Source: CAD feature listing. Evaluate the final solid. Frame: model axes, mm. A direction names the side the tool comes from. Give positions to 0.01 mm unless a question says otherwise; leave off trailing zeros. Order: outer loops, then holes, each group sorted by start corner. A loop starts at its lowest first (then second) coordinate and runs counter-clockwise, first axis right, second up. Notation, with made-up numbers: M -14,13.5 L 31,13.5 A21 ccw 31,40.5 Z; hole C -38.75,40.5 d9. An arc over 180 degrees is marked long. Answer in a Markdown table with one row per item. Add a question column.
(1) Set-up query: faces 5 (the face through (6.356, 8.801, 0.279)), 6 (the face through (15.12, 1.25, 11.59)). Return all of +Z, -Z, +X, -X, +Y, -Y with unobstructed straight access to the full face (end or side cutting, diameter ignored); none if empty.
(2) Section query A-A, the plane x = 0. Return loops of the section in (y, z).
(3) Section query C-C, the plane y = 8.5. Return loops of the section in (x, z), plus the area to 3 significant figures.
(4) Section query D-D, the plane z = -2.5. Return loops of the section in (x, y), plus the area to 3 significant figures.
(5) Section query B-B, the plane z = -9. Return loops of the section in (x, y), plus the area to 3 significant figures.
(6) Material intervals for line 1 along Y through (x, z) = (5, 7); line 2 along Z through (x, y) = (13, 14); line 3 along Z through (x, y) = (0, 2.5), sorted ascending.
(7) Pin query (flat end, axial travel): P1, Ø8, axis at y = 9.5, z = -3.5, coming from the -X side; P2, Ø4, axis at y = 7, z = -4.5, coming from the -X side; P3, Ø10, axis at y = 4.5, z = 13.5, coming from the -X side. Return the tip coordinate at first contact, or that it passes through.
(8) Mould query, pull axis Y, two halves, no side actions, for faces 1 (the face through (0, 0, 0)), 2 (the face through (-4, 2.54, 0)), 3 (the face through (0, 15.24, 0)), 4 (the face through (-15.12, 16.49, -11.59)). Classes: pulls with the +Y half, pulls with the -Y half, needs draft (parallel to the pull), parting line crosses it, or undercut.
Autodesk Inventor part; units mm, degrees
ref_plane "YZ Plane" through (0, 0, 0) normal (1, 0, 0) x (0, 1, 0)
ref_plane "XZ Plane" through (0, 0, 0) normal (0, 1, 0) x (-1, 0, 0)
ref_plane "XY Plane" through (0, 0, 0) normal (0, 0, 1) x (1, 0, 0)
sketch "Sketch1" plane through (0, 0, 0) normal (0, 1, 0) x (-1, 0, 0)
  circle A0 centre (0, 0) radius 19.05
  dimension "d0" = 38.1
extrude "Extrusion1" add sketch "Sketch1" along normal blind 2.54
sketch "Sketch2" plane through (0, 2.54, 0) normal (0, 1, 0) x (1, 0, 0)
  circle A0 centre (12.7, 0) radius 6.35
  point P0 (0, 0)
  dimension "d3" = 12.7
  dimension "d4" = 12.7
extrude "Extrusion2" add sketch "Sketch2" along normal blind 12.7
sketch "Sketch3" plane through (12.7, 15.24, 0) normal (0, 1, 0) x (1, 0, 0)
  circle A0 centre (-12.7, 0) radius 19.05
extrude "Extrusion3" add sketch "Sketch3" along normal blind 2.54
properties part number "ConcentricSupportTest1"
Values follow:
| question | item | result |
|---|---|---|
| 1 | face 5 | none |
| 1 | face 6 | +Y, -Y |
| 2 | outline | M 0,-19.05 L 2.54,-19.05 L 2.54,19.05 L 0,19.05 Z; M 15.24,-19.05 L 17.78,-19.05 L 17.78,19.05 L 15.24,19.05 Z |
| 3 | outline | C 12.7,0 d12.7 |
| 3 | area | 127 mm² |
| 4 | outline | M -18.89,0 L 18.89,0 L 18.89,2.54 L 18.54,2.54 L 18.54,15.24 L 18.89,15.24 L 18.89,17.78 L -18.89,17.78 L -18.89,15.24 L 6.86,15.24 L 6.86,2.54 L -18.89,2.54 Z |
| 4 | area | 340 mm² |
| 5 | outline | M -16.79,0 L 16.79,0 L 16.79,2.54 L -16.79,2.54 Z; M -16.79,15.24 L 16.79,15.24 L 16.79,17.78 L -16.79,17.78 Z |
| 5 | area | 171 mm² |
| 6 | line 1 | y = 0 to 2.54, 15.24 to 17.78 |
| 6 | line 2 | z = -6.34 to 6.34 |
| 6 | line 3 | z = -19.05 to 19.05 |
| 7 | P1 | stops at x = 6.35 |
| 7 | P2 | stops at x = 6.86 |
| 7 | P3 | stops at x = -16.84 |
| 8 | face 1 | pulls with the -Y half |
| 8 | face 2 | undercut |
| 8 | face 3 | undercut |
| 8 | face 4 | needs draft |
